Job drawing, mm, ordinate dimensions from the low corner. One solid piece. Give positions to 0.01 mm unless a question says otherwise; leave off trailing zeros. Order: outer loops, then holes, each group sorted by start corner. A loop starts at its lowest first (then second) coordinate and runs counter-clockwise, first axis right, second up.
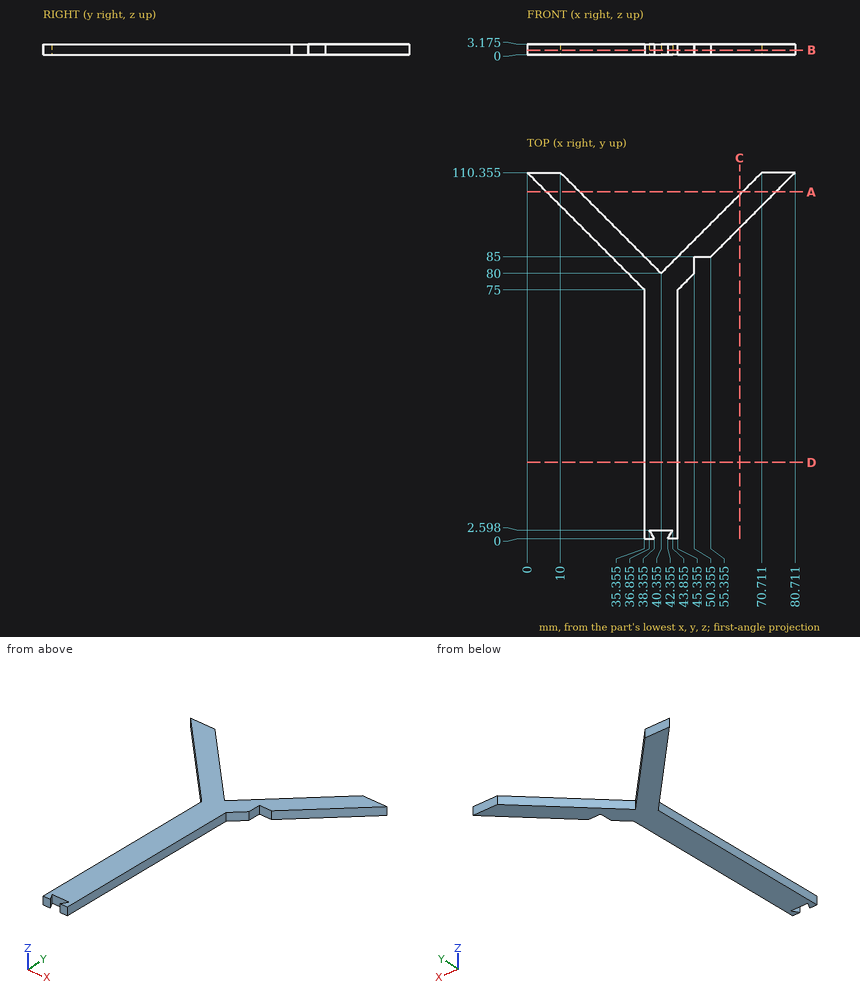
Item 1: Band-saw the part on D-D on y = 23. List the corners of the cut face in (x, z) (1 decimal).
Item 2: Drop flat-ended pins along their axis: P1, Ø1.6, axis at y = 82.5, z = 1.5, coming from the +X side (1 decimal); P2, Ø10, axis at x = 32.5, y = 13.5, coming from the +Z side (3 decimals); P3, Ø12, axis at x = 55.5, y = 69.5, coming from the -Z side; P4, Ø1.6, axis at x = 40.5, z = 2, coming from the -Y side. Give the stop position or say it passes through.
Item 3: Drill centre lines: probe 1 along X at (y, z) = (59.5, 2.3) (1 decimal); probe 2 along X at (y, z) = (86.5, 0.75) (1 decimal); probe 3 along Y at (x, z) = (10.5, 1.1) (1 decimal). Where is each one in solid material? Low to high.
Item 4: Band-saw the part on A-A on y = 104.5. List the corners of the cut face in (x, z) (1 decimal).
Item 5: Band-saw the part on C-C on x = 64. List the corners of the cut face in (y, z) (1 decimal).
Item 6: Band-saw the part on B-B on z = 1.3. List the corners of the cut face in (x, y) (1 decimal).
Working result:
1. outline: (35.4, 0) - (45.4, 0) - (45.4, 3.2) - (35.4, 3.2) - close
2. P1: stops at x = 50.4
2. P2: stops at z = 3.175
2. P3: passes through
2. P4: stops at y = 2.6
3. probe 1: x = 35.4 to 45.4
3. probe 2: x = 23.9 to 33.9, 46.9 to 56.9
3. probe 3: y = 99.9 to 109.9
4. outline: (5.9, 0) - (15.9, 0) - (15.9, 3.2) - (5.9, 3.2) - close; (64.9, 0) - (74.9, 0) - (74.9, 3.2) - (64.9, 3.2) - close
5. outline: (93.6, 0) - (103.6, 0) - (103.6, 3.2) - (93.6, 3.2) - close
6. outline: (0, 110.4) - (35.4, 75) - (35.4, 0) - (38.4, 0) - (36.9, 2.6) - (43.9, 2.6) - (42.4, 0) - (45.4, 0) - (45.4, 75) - (50.4, 80) - (50.4, 85) - (55.4, 85) - (80.7, 110.4) - (70.7, 110.4) - (40.4, 80) - (10, 110.4) - close
